from build123d import *

# Parameters (mm, degrees)
PAD_DEPTH    = 98
SKETCH001_R  = 5
POCKET_DEPTH = 25.001


with BuildPart() as part:
    # Sketch → Pad (new body)
    with BuildSketch(Plane.XZ):
        with BuildLine():
            Line((0, 0), (-25, 0))
            Line((-25, 0), (-25, 0.5))
            ThreePointArc((-21.5, 4), (-23.974874, 2.974874), (-25, 0.5))
            Line((-21.5, 4), (-7.5, 4))
            ThreePointArc((-7.5, 4), (-5.025126, 5.025126), (-4, 7.5))
            Line((-4, 7.5), (-4, 21.5))
            ThreePointArc((-0.5, 25), (-2.974874, 23.974874), (-4, 21.5))
            Line((-0.5, 25), (0, 25))
            Line((0, 25), (0, 0))
        make_face()
    extrude(amount=PAD_DEPTH)

    # Sketch001 → Pocket (cut, through all)
    with BuildSketch(Plane.XY):
        with Locations((-14.5, -10)):
            Circle(SKETCH001_R)
        with Locations((-14.5, -34)):
            Circle(SKETCH001_R)
        with Locations((-14.5, -88)):
            Circle(SKETCH001_R)
        with Locations((-14.5, -64)):
            Circle(SKETCH001_R)
    extrude(amount=POCKET_DEPTH, mode=Mode.SUBTRACT)


solid = part.part
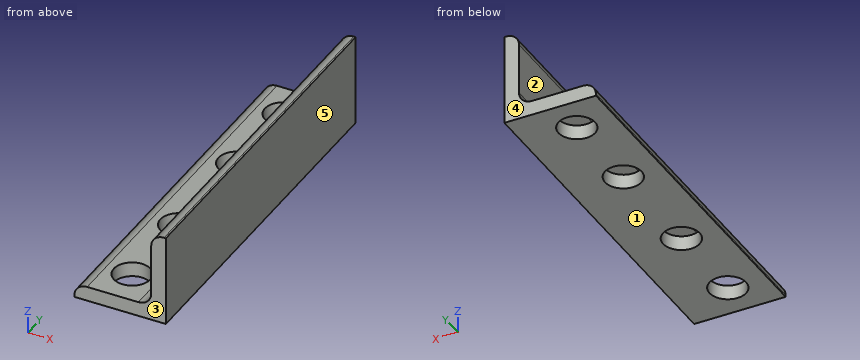
Verification items for the finished model (mm, model axes). Face numbers are marked on the shaded views. A direction names the side the tool comes from. Coordinates: 2 decimals unless noted, no trailing zeros. Order: outer loops, then holes, each group sorted by start corner. A loop starts at its lowest first (then second) coordinate and runs counter-clockwise, first axis right, second up. Notation, with made-up numbers: (36.5, 14.25) -> (73.5, 14.25) arc R19 ccw to (73.5, 46.25) -> close; hole circle Ø9 at (-35.75, 20). An arc over 180 degrees is marked (long way). Put each result on its own line as item: value. Start each with the question number.
1. Go/stop test with flat-tipped pins: pin 1 Ø7 at (y, z) = (-53, 14) entering from -X; pin 2 Ø1.5 at (x, y) = (-12, -29.5) entering from +Z; pin 3 Ø5 at (x, y) = (-5, -66) entering from +Z. Record where each tip stops, or that it passes through.
2. Cross-section at C-C, the plane z = 16.5. Record the boundary of the cut face in (x, y), then the cut area to 3 significant figures.
3. Material ranges on L1, parallel to Y at x = -14.5, z = 2.05; L2, parallel to X at y = -55.5, z = 8.5; L3, parallel to Z at x = -10, y = -67.5, recorded low to high. Write a range as [from, to].
4. Access from +Z, -Z, +X, -X, +Y, -Y to the whole of each face (thin tool, end or side, straight path). Record for the marked faces 1 and 2.
5. Cross-section at D-D, the plane y = -51. Record the boundary of the cut face in (x, z), then the cut area to 3 significant figures.
6. Cross-section at B-B, the plane y = -34. Record the boundary of the cut face in (x, z), then the cut area to 3 significant figures.
7. Mould release check, pull along Y, two halves, no side actions. Record for the marked faces 3, 4 and 5: released by +Y, released by -Y, zero draft, split by the parting line, or undercut.
8. Cross-section at A-A, the plane x = -14.5. Record the boundary of the cut face in (y, z).
Computed:
1. pin 1: x = -4
1. pin 2: z = 4
1. pin 3: z = 24.37
2. outline: (-4, -98) -> (0, -98) -> (0, 0) -> (-4, 0) -> close
2. area: 392 mm2
3. L1: [-98, -93], [-83, -69], [-59, -39], [-29, -15], [-5, 0]
3. L2: [-4, 0]
3. L3: [0, 4]
4. face 1: -Z, +X, -X, +Y, -Y
4. face 2: +Z, -X, +Y, -Y
5. outline: (-25, 0) -> (0, 0) -> (0, 25) -> (-0.5, 25) arc R3.5 ccw to (-4, 21.5) -> (-4, 7.5) arc R3.5 cw to (-7.5, 4) -> (-21.5, 4) arc R3.5 ccw to (-25, 0.5) -> close
5. area: 181 mm2
6. outline: (-25, 0) -> (-19.5, 0) -> (-19.5, 4) -> (-21.5, 4) arc R3.5 ccw to (-25, 0.5) -> close; (-9.5, 0) -> (0, 0) -> (0, 25) -> (-0.5, 25) arc R3.5 ccw to (-4, 21.5) -> (-4, 7.5) arc R3.5 cw to (-7.5, 4) -> (-9.5, 4) -> close
6. area: 141 mm2
7. face 3: released by -Y
7. face 4: released by +Y
7. face 5: zero draft
8. outline: (-98, 0) -> (-93, 0) -> (-93, 4) -> (-98, 4) -> close; (-83, 0) -> (-69, 0) -> (-69, 4) -> (-83, 4) -> close; (-59, 0) -> (-39, 0) -> (-39, 4) -> (-59, 4) -> close; (-29, 0) -> (-15, 0) -> (-15, 4) -> (-29, 4) -> close; (-5, 0) -> (0, 0) -> (0, 4) -> (-5, 4) -> close
